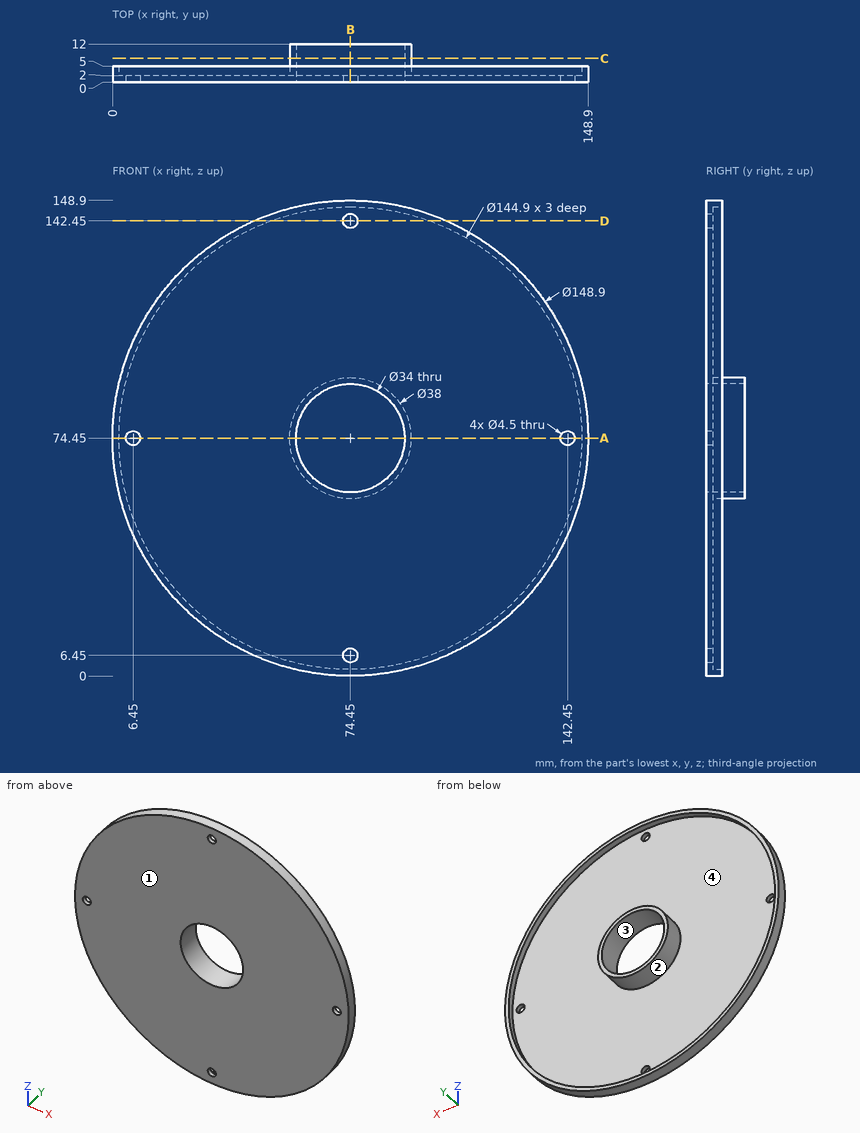
Geometry: see drawing. Coordinates: mm, zero at the bounding-box minimum. A direction names the side the tool comes from. Give positions to 0.01 mm unless a question says otherwise; leave off trailing zeros. Loops run counter-clockwise (first coordinate to the right, second up) from the corner with the lowest first, then second, coordinate; pieces in that order, holes last. Notation, with made-up numbers: M 83.25,44.25 L 119.25,44.25 A28 cw 119.25,68.25 Z; hole C 29.25,-12.75 d2. An arc over 180 degrees is marked long. Use one line per item in the form item = value.
1. Section query C-C, the plane y = 7.5. Return the cut outline in (x, z), and give its area (3 significant figures).
Numbers:
outline = C 74.45,74.45 d38; hole C 74.45,74.45 d34
area = 226 mm²
2. Reachability of the marked faces 3 and 4 from +Z, -Z, +X, -X, +Y, -Y: full face, straight path, thin tool, end or side. Return the list, or none.
Numbers:
face_3 = +Y, -Y
face_4 = +Y
3. Section query A-A, the plane z = 74.45. Return the cut outline in (x, y), and give its area (3 significant figures).
Numbers:
outline = M 0,0 L 4.2,0 L 4.2,2 L 2,2 L 2,5 L 0,5 Z; M 8.7,0 L 57.45,0 L 57.45,12 L 55.45,12 L 55.45,2 L 8.7,2 Z; M 91.45,0 L 140.2,0 L 140.2,2 L 93.45,2 L 93.45,12 L 91.45,12 Z; M 144.7,0 L 148.9,0 L 148.9,5 L 146.9,5 L 146.9,2 L 144.7,2 Z
area = 264 mm²
4. First-contact query: pin 1 (6 mm diameter, centred on x = 74.45, z = 142.45, fed in from -Y); pin 2 (5 mm diameter, centred on x = 93, y = 5, fed in from -Z); pin 3 (3.5 mm diameter, centred on x = 142.45, z = 74.45, fed in from +Y); pin 4 (8 mm diameter, centred on x = 57.5, z = 32, fed in from +Y). Flat tips, straight axial feed; report the tip coordinate or a pass-through.
Numbers:
pin_1 = 0
pin_2 = 1.75
pin_3 = through
pin_4 = 2
5. Pull-direction query (X, two-part tool) for the marked faces 1 and 2; classes: released by +X, released by -X, zero draft, split by the parting line, or undercut.
Numbers:
face_1 = zero draft
face_2 = undercut
6. Section query B-B, the plane x = 74.45. Return the cut outline in (y, z).
Numbers:
outline = M 0,0 L 5,0 L 5,2 L 2,2 L 2,4.2 L 0,4.2 Z; M 0,8.7 L 2,8.7 L 2,55.45 L 12,55.45 L 12,57.45 L 0,57.45 Z; M 0,91.45 L 12,91.45 L 12,93.45 L 2,93.45 L 2,140.2 L 0,140.2 Z; M 0,144.7 L 2,144.7 L 2,146.9 L 5,146.9 L 5,148.9 L 0,148.9 Z
7. Section query D-D, the plane z = 142.45. Return the cut outline in (x, y), and give its area (3 significant figures).
Numbers:
outline = M 44.14,0 L 72.2,0 L 72.2,2 L 49.45,2 L 49.45,5 L 44.14,5 Z; M 76.7,0 L 104.76,0 L 104.76,5 L 99.45,5 L 99.45,2 L 76.7,2 Z
area = 144 mm²
8. Line query: L1, parallel to X at y = 1.2, z = 74.45; L2, parallel to X at y = 2.9, z = 74.45; L3, parallel to Z at x = 85, y = 3.5. Output: solid intervals per line, ascending.
Numbers:
L1 = 0 to 4.2, 8.7 to 57.45, 91.45 to 140.2, 144.7 to 148.9
L2 = 0 to 2, 55.45 to 57.45, 91.45 to 93.45, 146.9 to 148.9
L3 = 0.75 to 2.77, 58.65 to 61.12, 87.78 to 90.25, 146.13 to 148.15
